Source: CAD feature listing. Evaluate the final solid. Frame: model axes, mm. Round coordinates to 2 decimals unless told otherwise and drop trailing zeros. Loops run counter-clockwise (first coordinate to the right, second up) from the corner with the lowest first, then second, coordinate; pieces in that order, holes last.
(1) Section A-A, the plane x = -3. Return the cut outline in (y, z).
(2) Section B-B, the plane z = 361. Count the separate pieces of the cut face and the enclosed holes in it, plus the area to 3 significant figures.
(3) First-contact query: pin 1 Ø3.5 at (x, z) = (20.5, 255) entering from +Y; pin 2 Ø1 at (y, z) = (-1.5, 198) entering from -X. Flat tips, straight axial feed; report the tip coordinate or a pass-through.
(4) Material intervals for probe 1 along X at (y, z) = (-4.5, 160.5); probe 2 along X at (y, z) = (-14.5, 390); probe 3 along Y at (x, z) = (-34, 94.5), sorted ascending.
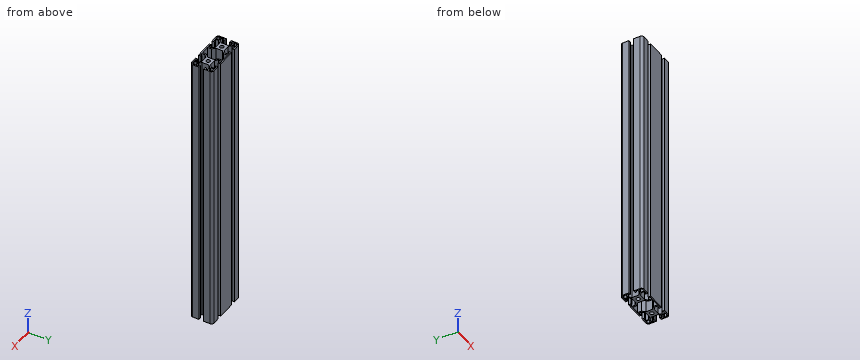
```python
from build123d import *

# Parameters (mm, degrees)
SKETCH1_R           = 3.4
BOSS_EXTRUDE1_DEPTH = 500


with BuildPart() as part:
    # Sketch1 → Boss-Extrude1 (new body)
    with BuildSketch(Plane.XY):
        with BuildLine():
            Line((24.1, -20), (35.5, -20))
            ThreePointArc((35.5, -20), (38.681980515, -18.681980515), (40, -15.5))
            Line((40, -15.5), (40, -4.1))
            Line((40, -4.1), (35.5, -4.1))
            Line((35.5, -4.1), (35.5, -6.6))
            Line((35.5, -6.6), (38, -6.6))
            Line((38, -6.6), (38, -10.25))
            Line((38, -10.25), (32.017766953, -10.25))
            Line((32.017766953, -10.25), (27.7, -5.932233047))
            Line((27.7, -5.932233047), (27.7, 5.932233047))
            Line((27.7, 5.932233047), (32.017766953, 10.25))
            Line((32.017766953, 10.25), (38, 10.25))
            Line((38, 10.25), (38, 6.6))
            Line((38, 6.6), (35.5, 6.6))
            Line((35.5, 6.6), (35.5, 4.1))
            Line((35.5, 4.1), (40, 4.1))
            Line((40, 4.1), (40, 15.5))
            ThreePointArc((40, 15.5), (38.681980515, 18.681980515), (35.5, 20))
            Line((35.5, 20), (24.1, 20))
            Line((24.1, 20), (24.1, 15.5))
            Line((24.1, 15.5), (26.6, 15.5))
            Line((26.6, 15.5), (26.6, 18))
            Line((26.6, 18), (30.25, 18))
            Line((30.25, 18), (30.25, 12.017766953))
            Line((30.25, 12.017766953), (25.932233047, 7.7))
            Line((25.932233047, 7.7), (14.067766953, 7.7))
            Line((14.067766953, 7.7), (9.75, 12.017766953))
            Line((9.75, 12.017766953), (9.75, 18))
            Line((9.75, 18), (13.4, 18))
            Line((13.4, 18), (13.4, 15.5))
            Line((13.4, 15.5), (15.9, 15.5))
            Line((15.9, 15.5), (15.9, 20))
            Line((15.9, 20), (-15.9, 20))
            Line((-15.9, 20), (-15.9, 15.5))
            Line((-15.9, 15.5), (-13.4, 15.5))
            Line((-13.4, 15.5), (-13.4, 18))
            Line((-13.4, 18), (-9.75, 18))
            Line((-9.75, 18), (-9.75, 12.017766953))
            Line((-9.75, 12.017766953), (-14.067766953, 7.7))
            Line((-14.067766953, 7.7), (-25.932233047, 7.7))
            Line((-25.932233047, 7.7), (-30.25, 12.017766953))
            Line((-30.25, 12.017766953), (-30.25, 18))
            Line((-30.25, 18), (-26.6, 18))
            Line((-26.6, 18), (-26.6, 15.5))
            Line((-26.6, 15.5), (-24.1, 15.5))
            Line((-24.1, 15.5), (-24.1, 20))
            Line((-24.1, 20), (-35.5, 20))
            ThreePointArc((-35.5, 20), (-38.681980515, 18.681980515), (-40, 15.5))
            Line((-40, 15.5), (-40, 4.1))
            Line((-40, 4.1), (-35.5, 4.1))
            Line((-35.5, 4.1), (-35.5, 6.6))
            Line((-35.5, 6.6), (-38, 6.6))
            Line((-38, 6.6), (-38, 10.25))
            Line((-38, 10.25), (-32.017766953, 10.25))
            Line((-32.017766953, 10.25), (-27.7, 5.932233047))
            Line((-27.7, 5.932233047), (-27.7, -5.932233047))
            Line((-27.7, -5.932233047), (-32.017766953, -10.25))
            Line((-32.017766953, -10.25), (-38, -10.25))
            Line((-38, -10.25), (-38, -6.6))
            Line((-38, -6.6), (-35.5, -6.6))
            Line((-35.5, -6.6), (-35.5, -4.1))
            Line((-35.5, -4.1), (-40, -4.1))
            Line((-40, -4.1), (-40, -15.5))
            ThreePointArc((-40, -15.5), (-38.681980515, -18.681980515), (-35.5, -20))
            Line((-35.5, -20), (-24.1, -20))
            Line((-24.1, -20), (-24.1, -15.5))
            Line((-24.1, -15.5), (-26.6, -15.5))
            Line((-26.6, -15.5), (-26.6, -18))
            Line((-26.6, -18), (-30.25, -18))
            Line((-30.25, -18), (-30.25, -12.017766953))
            Line((-30.25, -12.017766953), (-25.932233047, -7.7))
            Line((-25.932233047, -7.7), (-14.067766953, -7.7))
            Line((-14.067766953, -7.7), (-9.75, -12.017766953))
            Line((-9.75, -12.017766953), (-9.75, -18))
            Line((-9.75, -18), (-13.4, -18))
            Line((-13.4, -18), (-13.4, -15.5))
            Line((-13.4, -15.5), (-15.9, -15.5))
            Line((-15.9, -15.5), (-15.9, -20))
            Line((-15.9, -20), (15.9, -20))
            Line((15.9, -20), (15.9, -15.5))
            Line((15.9, -15.5), (13.4, -15.5))
            Line((13.4, -15.5), (13.4, -18))
            Line((13.4, -18), (9.75, -18))
            Line((9.75, -18), (9.75, -12.017766953))
            Line((9.75, -12.017766953), (14.067766953, -7.7))
            Line((14.067766953, -7.7), (25.932233047, -7.7))
            Line((25.932233047, -7.7), (30.25, -12.017766953))
            Line((30.25, -12.017766953), (30.25, -18))
            Line((30.25, -18), (26.6, -18))
            Line((26.6, -18), (26.6, -15.5))
            Line((26.6, -15.5), (24.1, -15.5))
            Line((24.1, -15.5), (24.1, -20))
        make_face()
        with Locations((-20, 0)):
            Circle(SKETCH1_R, mode=Mode.SUBTRACT)
        with Locations((20, 0)):
            Circle(SKETCH1_R, mode=Mode.SUBTRACT)
        with BuildLine():
            Line((38, -15.5), (38, -11.75))
            Line((38, -11.75), (31.75, -11.75))
            Line((31.75, -11.75), (31.75, -18))
            Line((31.75, -18), (35.5, -18))
            ThreePointArc((35.5, -18), (37.267766953, -17.267766953), (38, -15.5))
        make_face(mode=Mode.SUBTRACT)
        with BuildLine():
            Line((-38, 15.5), (-38, 11.75))
            Line((-38, 11.75), (-31.75, 11.75))
            Line((-31.75, 11.75), (-31.75, 18))
            Line((-31.75, 18), (-35.5, 18))
            ThreePointArc((-35.5, 18), (-37.267766953, 17.267766953), (-38, 15.5))
        make_face(mode=Mode.SUBTRACT)
        Polygon((-7.25, -10.982233047), (-7.25, -17.8), (7.25, -17.8), (7.25, -10.982233047), (12.3, -5.932233047), (12.3, 5.932233047), (7.25, 10.982233047), (7.25, 17.8), (-7.25, 17.8), (-7.25, 10.982233047), (-12.3, 5.932233047), (-12.3, -5.932233047), align=None, mode=Mode.SUBTRACT)
        with BuildLine():
            Line((-35.5, -18), (-31.75, -18))
            Line((-31.75, -18), (-31.75, -11.75))
            Line((-31.75, -11.75), (-38, -11.75))
            Line((-38, -11.75), (-38, -15.5))
            ThreePointArc((-38, -15.5), (-37.267766953, -17.267766953), (-35.5, -18))
        make_face(mode=Mode.SUBTRACT)
        with BuildLine():
            Line((35.5, 18), (31.75, 18))
            Line((31.75, 18), (31.75, 11.75))
            Line((31.75, 11.75), (38, 11.75))
            Line((38, 11.75), (38, 15.5))
            ThreePointArc((38, 15.5), (37.267766953, 17.267766953), (35.5, 18))
        make_face(mode=Mode.SUBTRACT)
    extrude(amount=BOSS_EXTRUDE1_DEPTH)


solid = part.part
```
Output values:
1. outline: (-20, 0) - (-17.8, 0) - (-17.8, 500) - (-20, 500) - close; (17.8, 0) - (20, 0) - (20, 500) - (17.8, 500) - close
2. separate pieces: 1
2. enclosed holes: 7
2. area: 1,090 mm2
3. pin 1: stops at y = 7.7
3. pin 2: stops at x = -27.7
4. probe 1: x = -40 to -35.5, -27.7 to -12.3, 12.3 to 27.7, 35.5 to 40
4. probe 2: x = -40 to -38, -31.75 to -30.25, -9.75 to -7.25, 7.25 to 9.75, 30.25 to 31.75, 38 to 40
4. probe 3: y = -20 to -18, -11.75 to -10.25, 10.25 to 11.75, 18 to 20
